from build123d import *

# Parameters (mm, degrees)
IZIM2_R                     = 1.75
Y_KSEKLIK_EKSTR_ZYON1_DEPTH = 2
PAH1_SIZE                   = 1
IZIM3_W                     = 10
IZIM3_H                     = 1.5
KES_EKSTR_ZYON1_DEPTH       = 10


with BuildPart() as part:
    # Çizim2 → Yükseklik-Ekstrüzyon1 (new body)
    with BuildSketch(Plane(origin=(0, 0, 0), x_dir=(1, 0, 0), z_dir=(0, 1, 0))):
        with BuildLine():
            Line((19.655461919, 42.650157531), (32.155461919, 7.650157531))
            ThreePointArc((32.155461919, 7.650157531), (31.658156515, 4.000618196), (28.388494273, 2.304811943))
            Line((28.388494273, 2.304811943), (4.365814172, 2.304811943))
            ThreePointArc((4.365814172, 2.304811943), (0.022651908, 3.932838217), (-0.04976512, 8.570540641))
            Line((-0.04976512, 8.570540641), (12.121526627, 42.650157531))
            ThreePointArc((12.121526627, 42.650157531), (15.888494273, 45.304811943), (19.655461919, 42.650157531))
        make_face()
        with Locations(Location((3.388494273, 6.304811943, 0), (0, 0, 270))):
            Circle(IZIM2_R, mode=Mode.SUBTRACT)
        with Locations(Location((28.388494273, 6.304811943, 0), (0, 0, 270))):
            Circle(IZIM2_R, mode=Mode.SUBTRACT)
        with Locations(Location((15.888494273, 41.304811943, 0), (0, 0, 270))):
            Circle(IZIM2_R, mode=Mode.SUBTRACT)
        with BuildLine():
            Line((14.543148685, 37.537844297), (4.733839861, 10.07177959))
            ThreePointArc((4.733839861, 10.07177959), (6.658156515, 8.60900569), (7.388494273, 6.304811943))
            Line((7.388494273, 6.304811943), (24.388494273, 6.304811943))
            ThreePointArc((24.388494273, 6.304811943), (25.118832031, 8.60900569), (27.043148685, 10.07177959))
            Line((27.043148685, 10.07177959), (17.233839861, 37.537844297))
            ThreePointArc((17.233839861, 37.537844297), (15.888494273, 37.304811943), (14.543148685, 37.537844297))
        make_face(mode=Mode.SUBTRACT)
    extrude(amount=Y_KSEKLIK_EKSTR_ZYON1_DEPTH)

    # Pah1
    pah1_edges = [part.edges().sort_by_distance(p)[0] for p in [
        (3.388494273, 2, -8.054811943),
        (28.388494273, 2, -8.054811943),
        (15.888494273, 2, -43.054811943),
    ]]
    chamfer(pah1_edges, length=PAH1_SIZE)

    # Çizim3 → Kes-Ekstrüzyon1 (cut)
    with BuildSketch(Plane(origin=(0, 2, 0), x_dir=(1, 0, 0), z_dir=(0, 1, 0))):
        with Locations((15.888494273, 44.554811943)):
            Rectangle(IZIM3_W, IZIM3_H)
    extrude(amount=-KES_EKSTR_ZYON1_DEPTH, mode=Mode.SUBTRACT)


solid = part.part
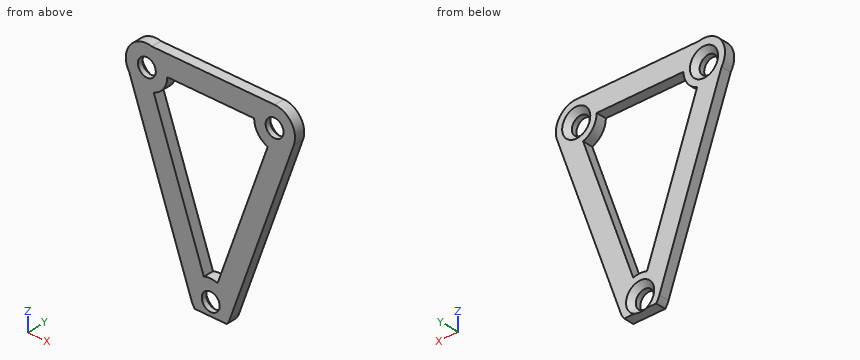
Geometry: final body of the model. Coordinates: model frame, mm. Coordinates: 2 decimals unless noted, no trailing zeros. Order: outer loops, then holes, each group sorted by start corner. A loop starts at its lowest first (then second) coordinate and runs counter-clockwise, first axis right, second up.
(1) Section query B-B (z = -23). Return the cut outline in (x, y).
(2) Section query A-A (x = 23). Return the cut outline in (y, z), plus the area to 3 significant figures.
(3) Section query C-C (y = 1.3). Return the cut outline in (x, z).
(4) First-contact query: pin 1 (2 mm diameter, centred on x = 28.39, z = -6.3, fed in from -Y); pin 2 (4.5 mm diameter, centred on x = 3.39, z = -6.3, fed in from +Y); pin 3 (4 mm diameter, centred on x = 15.89, z = -41.3, fed in from +Y). Flat tips, straight axial feed; report the tip coordinate or a pass-through.
(5) Material intervals for probe 1 along X at (y, z) = (0.7, -18); probe 2 along X at (y, z) = (1.85, -21), sorted ascending.
(6) Section query D-D (z = -5.5). State how many separate pieces and enclosed holes the cut face has, plus the area to 3 significant figures.
Solution:
1. outline: (5.1, 0) - (9.35, 0) - (9.35, 2) - (5.1, 2) - close; (22.43, 0) - (26.67, 0) - (26.67, 2) - (22.43, 2) - close
2. outline: (0, -33.29) - (2, -33.29) - (2, -21.39) - (0, -21.39) - close; (0, -6.3) - (2, -6.3) - (2, -2.3) - (0, -2.3) - close
2. area: 31.8 mm2
3. outline: (-0.05, -8.57) - (12.12, -42.65) arc R4 ccw to (12.77, -43.8) - (19.01, -43.8) arc R4 ccw to (19.66, -42.65) - (32.16, -7.65) arc R4 ccw to (28.39, -2.3) - (4.37, -2.3) arc R4.12 ccw to start; hole circle Ø4.1 at (3.39, -6.3); hole (4.73, -10.07) - (14.54, -37.54) arc R4 cw to (17.23, -37.54) - (27.04, -10.07) arc R4 cw to (24.39, -6.3) - (7.39, -6.3) arc R4 cw to start; hole circle Ø4.1 at (15.89, -41.3); hole circle Ø4.1 at (28.39, -6.3)
4. pin 1: passes through
4. pin 2: stops at y = 1.51
4. pin 3: stops at y = 1.26
5. probe 1: x = 3.32 to 7.57, 24.21 to 28.46
5. probe 2: x = 4.39 to 8.64, 23.14 to 27.39
6. separate pieces: 3
6. enclosed holes: 0
6. area: 51.3 mm2
